Part print with two shaded views. Sizes in mm from the minimum x, y, z corner. A direction names the side the tool comes from. Round coordinates to 2 decimals unless told otherwise and drop trailing zeros. Loops run counter-clockwise (first coordinate to the right, second up) from the corner with the lowest first, then second, coordinate; pieces in that order, holes last.
(1) Cut at C-C on y = 9.5. List the corners of the cut face in (x, z), then the cut area to 3 significant figures.
(2) Tool access for the marked faces 1 and 2: list every direction of +Z, -Z, +X, -X, +Y, -Y with a clear straight run to the whole face (end or side of a thin tool).
(3) Cut at B-B on z = 16.5. List the corners of the cut face in (x, y), then the cut area to 3 significant figures.
(4) Flat gauge pins, fed straight in: pin 1 (1 mm diameter, centred on y = 7.5, z = 13.5, fed in from +X); pin 2 (1.8 mm diameter, centred on y = 10.5, z = 17.5, fed in from +X). Where does each tip first touch, or does it go through?
(5) Probe probe 1 along Y at (x, z) = (24.75, 22.75); probe 2 along X at (y, z) = (8.25, 11.25); probe 3 along Y at (x, z) = (6.5, 16.5). List the from-to ranges inside material, lowest first.
(6) Cut at A-A on x = 8.75. List the corners of the cut face in (y, z).
(7) Mould opens along Y. For the marked faces 3, 4 and 5 say: +Y half, -Y half, draft (parallel to the pull), parting line (faces both ways), or undercut.
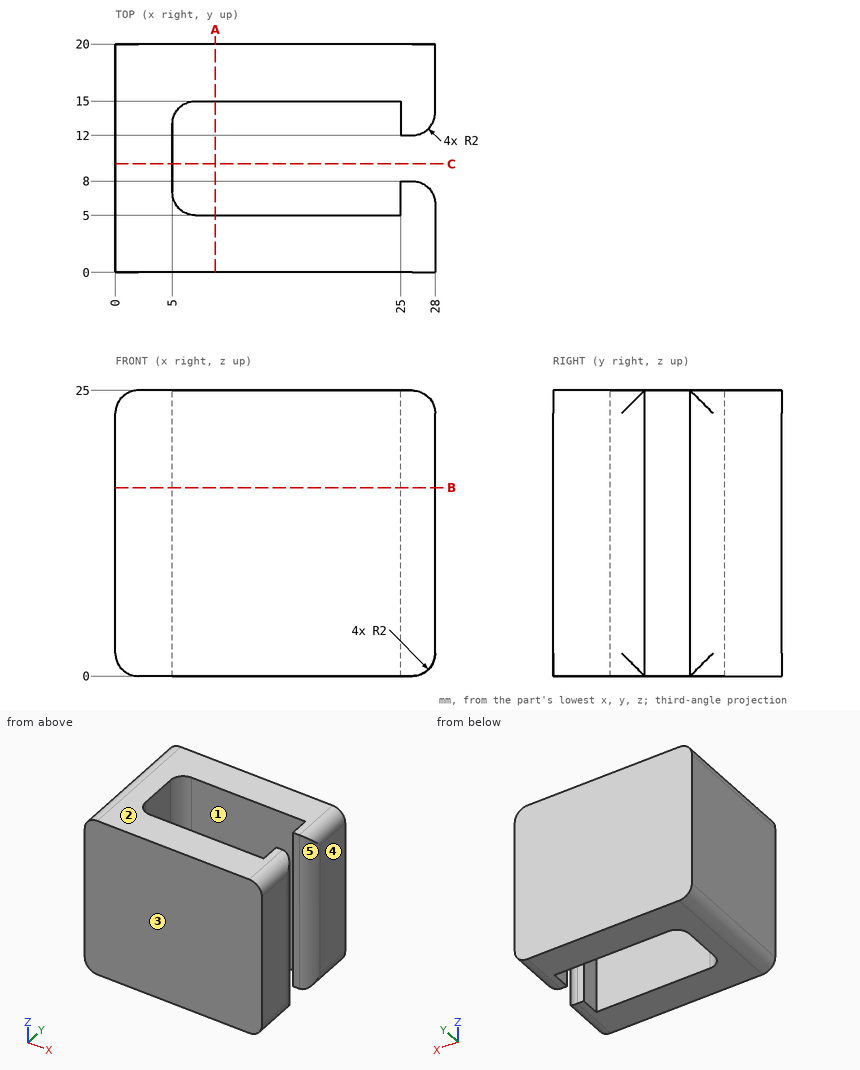
Final values:
1. outline: (0, 2) arc R2 ccw to (2, 0) - (5, 0) - (5, 25) - (2, 25) arc R2 ccw to (0, 23) - close
1. area: 123 mm2
2. face 1: +Z, -Z
2. face 2: +Z, +X, -X, +Y, -Y
3. outline: (0, 0) - (28, 0) - (28, 6) arc R2 ccw to (26, 8) - (25, 8) - (25, 5) - (7, 5) arc R2 cw to (5, 7) - (5, 13) arc R2 cw to (7, 15) - (25, 15) - (25, 12) - (26, 12) arc R2 ccw to (28, 14) - (28, 20) - (0, 20) - close
3. area: 348 mm2
4. pin 1: stops at x = 27.73
4. pin 2: stops at x = 5
5. probe 1: y = 0 to 5, 15 to 20
5. probe 2: x = 0 to 5
5. probe 3: y = 0 to 5.06, 14.94 to 20
6. outline: (0, 0) - (5, 0) - (5, 25) - (0, 25) - close; (15, 0) - (20, 0) - (20, 25) - (15, 25) - close
7. face 3: -Y half
7. face 4: draft
7. face 5: undercut
